from build123d import *

# Parameters (mm, degrees)
F0_R     = 4.699
F0_R_2   = 3.302
F1_DEPTH = 4.7625


with BuildPart() as f1:
    # F0 (on Front) → F1 (new body)
    with BuildSketch(Plane.XZ):
        with BuildLine():
            Line((0, 12.7), (0, 10.292423))
            ThreePointArc((0, 10.292423), (1.394452, 6.3219), (4.965369, 4.095222))
            Line((4.965369, 4.095222), (98.498426, -16.80273))
            ThreePointArc((98.498426, -16.80273), (102.208704, -17.13197), (105.877239, -16.48667))
            Line((105.877239, -16.48667), (124.088291, -10.744747))
            ThreePointArc((124.088291, -10.744747), (133.377536, -1.453733), (131.09241, 11.484244))
            Line((131.09241, 11.484244), (111.773368, 36.641459))
            ThreePointArc((111.773368, 36.641459), (106.399109, 40.724398), (99.696147, 41.513923))
            Line((99.696147, 41.513923), (5.407499, 27.362341))
            ThreePointArc((5.407499, 27.362341), (1.538172, 25.226203), (0, 21.082676))
            Line((0, 21.082676), (0, 19.304))
            Line((0, 19.304), (12.7, 19.304))
            Line((12.7, 19.304), (12.7, 12.7))
            Line((12.7, 12.7), (0, 12.7))
        make_face()
        with Locations((101.6, -2.921)):
            Circle(F0_R, mode=Mode.SUBTRACT)
        with Locations((119.811052, 2.820923)):
            Circle(F0_R, mode=Mode.SUBTRACT)
        with Locations((101.6, 28.829)):
            Circle(F0_R_2, mode=Mode.SUBTRACT)
    extrude(amount=F1_DEPTH)


solid = f1.part
Geometry: final body of the model. Coordinates: model frame, mm. A direction names the side the tool comes from. Round coordinates to 2 decimals unless told otherwise and drop trailing zeros. Loops run counter-clockwise (first coordinate to the right, second up) from the corner with the lowest first, then second, coordinate; pieces in that order, holes last. Notation, with made-up numbers: M 0,-19.5 L 19,-19.5 A29 ccw 19,8.5 Z; hole C -34,75 d2. An arc over 180 degrees is marked long. One line per question, with ' | ' between items.
(1) Cut plane B-B on z = 5.5. Return the cut outline in (x, y).
Check result:
outline: M 2.18,-4.76 L 115.95,-4.76 L 115.95,0 L 2.18,0 Z; M 123.67,-4.76 L 133.78,-4.76 L 133.78,0 L 123.67,0 Z
(2) Cut plane A-A on x = 101.6. Return the cut outline in (y, z) (1 decimal), plus the area to 3 significant figures.
Check result:
outline: M -4.8,-17.1 L 0,-17.1 L 0,-7.6 L -4.8,-7.6 Z; M -4.8,1.8 L 0,1.8 L 0,25.5 L -4.8,25.5 Z; M -4.8,32.1 L 0,32.1 L 0,41.7 L -4.8,41.7 Z | area: 204 mm2
(3) Pull-direction query (Z, two-part tool) for faces 3 (the flat face through (51.08, -2.35, -6.21)), 4 (the cylindrical face through (106.488, -2.348, 40.688)), 5 (the cylindrical face through (106.082, -2.348, -1.51)); classes: +Z half, -Z half, draft (parallel to the pull), parting line (faces both ways), or undercut.
Check result:
face 3: -Z half | face 4: +Z half | face 5: undercut
(4) Material intervals for line 1 along Z through (x, y) = (101.6, -2.9) (3 decimals); line 2 along X through (y, z) = (-3.4, 6.5); line 3 along X through (y, z) = (-0.4, 14), sorted ascending. Write a range as from..to.
Check result:
line 1: z = -17.145..-7.62, 1.778..25.527, 32.131..41.656 | line 2: x = 1.26..116.89, 122.73..133.55 | line 3: x = 12.7..129.16
(5) Contact query for flat-ended pins moving along their axis: P1, Ø1.4, axis at x = 3.5, y = -1, coming from the +Z side; P2, Ø2, axis at x = 89, y = -1.5, coming from the +Z side; P3, Ø2.5, axis at y = -2.5, z = 16.5, coming from the -X side. Output: stop coordinate, or through.
Check result:
P1: stops at z = 27.06 | P2: stops at z = 40.06 | P3: stops at x = 12.7
(6) Access query for faces 1 (the flat face through (6, -2, 19.304)), 2 (the cylindrical face through (133.319, -2.348, -1.636)). Directions: +Z, -Z, +X, -X, +Y, -Y. A direction counts if a zero-diameter tool reaches every point of the face in a straight line with its end or side. Return the directions, or none.
Check result:
face 1: -X, +Y, -Y | face 2: +X, +Y, -Y
(7) Cut plane D-D on z = 38. Return the cut outline in (x, y), plus the area to 3 significant figures.
Check result:
outline: M 76.28,-4.76 L 110.57,-4.76 L 110.57,0 L 76.28,0 Z | area: 163 mm2
(8) Cut plane C-C on y = -2.5. Return the cut outline in (x, z), plus the area to 3 significant figures.
Check result:
outline: M 0,10.29 A6.35 ccw 4.97,4.1 L 98.5,-16.8 A14.22 ccw 105.88,-16.49 L 124.09,-10.74 A14.22 ccw 131.09,11.48 L 111.77,36.64 A12.83 ccw 99.7,41.51 L 5.41,27.36 A6.35 ccw 0,21.08 L 0,19.3 L 12.7,19.3 L 12.7,12.7 L 0,12.7 Z; hole C 101.6,-2.92 d9.4; hole C 101.6,28.83 d6.6; hole C 119.81,2.82 d9.4 | area: 5,120 mm2
